from build123d import *

# Parameters (mm, degrees)
SKETCH1_R           = 4
SKETCH1_R_2         = 1.9
BOSS_EXTRUDE1_DEPTH = 2


with BuildPart() as part:
    # Sketch1 → Boss-Extrude1 (new body)
    # profile 1 of 4: a face of its own
    with BuildSketch(Plane(origin=(0, 0, 0), x_dir=(1, 0, 0), z_dir=(0, 1, 0))):
        with Locations((-6.8, 4)):
            Circle(SKETCH1_R)
        with Locations(Location((-6.8, 4, 0), (0, 0, 270))):
            Circle(SKETCH1_R_2, mode=Mode.SUBTRACT)
    # profile 2 of 4: a face of its own
    with BuildSketch(Plane(origin=(0, 0, 0), x_dir=(1, 0, 0), z_dir=(0, 1, 0))):
        with BuildLine():
            Line((-6.8, 0), (0, 0))
            Line((0, 0), (0, 4.5))
            Line((0, 4.5), (-2.831373033, 4.5))
            ThreePointArc((-2.831373033, 4.5), (-2.807850963, 4.25049165), (-2.8, 4))
            ThreePointArc((-2.8, 4), (-3.971572875, 1.171572875), (-6.8, 0))
        make_face()
    # profile 3 of 4: a face of its own
    with BuildSketch(Plane(origin=(0, 0, 0), x_dir=(1, 0, 0), z_dir=(0, 1, 0))):
        with BuildLine():
            Line((0, 4.5), (0, 0))
            Line((0, 0), (6.8, 0))
            ThreePointArc((6.8, 0), (3.8, 1.354248689), (2.831373033, 4.5))
            Line((2.831373033, 4.5), (0, 4.5))
        make_face()
    # profile 4 of 4: a face of its own
    with BuildSketch(Plane(origin=(0, 0, 0), x_dir=(1, 0, 0), z_dir=(0, 1, 0))):
        with Locations((6.8, 4)):
            Circle(SKETCH1_R)
        with Locations(Location((6.8, 4, 0), (0, 0, 270))):
            Circle(SKETCH1_R_2, mode=Mode.SUBTRACT)
    extrude(amount=BOSS_EXTRUDE1_DEPTH)


solid = part.part
Source: CAD feature listing. Evaluate the final solid. Frame: model axes, mm. Give positions to 0.01 mm unless a question says otherwise; leave off trailing zeros. Write each loop counter-clockwise with the first axis right and the second up, starting at its lowest first coordinate (ties: lowest second). Pieces come first, ordered by that corner, then holes. Notation, with made-up numbers: M 25.5,19 L 72.5,19 A28 cw 72.5,54 Z; hole C 74.25,-5 d8. An arc over 180 degrees is marked long. Return JSON: item names as keys, results as strings. Group by question number.
1) First-contact query: pin 1 Ø4 at (x, z) = (7, -5.5) entering from +Y. Flat tip, straight axial feed; report the tip coordinate or a pass-through.
2) Ray query, L1, parallel to X at y = 0.7, z = -4; L2, parallel to Z at x = -8, y = 0.7; L3, parallel to Z at x = -6, y = 0.95. Return the intervals inside material, ascending.
3) Draft query along Z for faces 1 (the face through (0, 1, -4.5)), 2 (the face through (5.644, 0.986, -5.508)), 3 (the face through (-5.516, 0.986, -5.4)), 4 (the face through (9.88, 0.99, -6.55)). Return one class per face: released by +Z, released by -Z, zero draft, split by the parting line, or undercut.
4) Cut plane C-C, the plane y = 1.1. Output: boundary loops of the cut face in (x, z), then the cut area to 3 significant figures.
5) Cut plane D-D, the plane z = -5. Output: boundary loops of the cut face in (x, y), then the cut area to 3 significant figures.
6) Cut plane B-B, the plane x = 7.5. Output: boundary loops of the cut face in (y, z), then the cut area to 3 significant figures.
7) Cut plane A-A, the plane z = -4. Output: boundary loops of the cut face in (x, y).
Data:
{
 "1": {"pin 1": "stops at y = 2"},
 "2": {"L1": "x = -10.8 to -8.7, -4.9 to 4.9, 8.7 to 10.8", "L2": "z = -7.82 to -5.47, -2.53 to -0.18", "L3": "z = -7.92 to -5.72, -2.28 to 0"},
 "3": {"face 1": "released by -Z", "face 2": "undercut", "face 3": "undercut", "face 4": "split by the parting line"},
 "4": {"outline": "M -6.8,0 A4 ccw long -2.83,-4.5 L 2.83,-4.5 A4 ccw long 6.8,0 Z; hole C -6.8,-4 d3.8; hole C 6.8,-4 d3.8", "area": "110 mm²"},
 "5": {"outline": "M -10.67,0 L -8.42,0 L -8.42,2 L -10.67,2 Z; M -5.18,0 L -2.93,0 L -2.93,2 L -5.18,2 Z; M 2.93,0 L 5.18,0 L 5.18,2 L 2.93,2 Z; M 8.42,0 L 10.67,0 L 10.67,2 L 8.42,2 Z", "area": "18.1 mm²"},
 "6": {"outline": "M 0,-7.94 L 2,-7.94 L 2,-5.77 L 0,-5.77 Z; M 0,-2.23 L 2,-2.23 L 2,-0.06 L 0,-0.06 Z", "area": "8.69 mm²"},
 "7": {"outline": "M -10.8,0 L -8.7,0 L -8.7,2 L -10.8,2 Z; M -4.9,0 L 4.9,0 L 4.9,2 L -4.9,2 Z; M 8.7,0 L 10.8,0 L 10.8,2 L 8.7,2 Z"}
}
